Can you work these out from the model? Positions are in its coordinate system, mm. Face numbers are marked on the shaded views. A direction names the side the tool comes from. Coordinates: 2 decimals unless noted, no trailing zeros. Write each loop counter-clockwise with the first axis right and the second up, starting at its lowest first coordinate (ties: lowest second). Pieces come first, ordered by that corner, then holes.
```python
from build123d import *

# Parameters (mm, degrees)
SKETCH1_R           = 5
SKETCH1_R_2         = 1.8
BOSS_EXTRUDE1_DEPTH = 10
CHAMFER1_SIZE       = 0.5
CUT_EXTRUDE2_DEPTH  = 2.5
CHAMFER2_SIZE       = 0.5
SKETCH4_R           = 1.8
CUT_EXTRUDE3_DEPTH  = 10
CHAMFER3_SIZE       = 0.5
CHAMFER3_SIZE_2     = 0.923879533
CHAMFER3_SIZE_3     = 0.552958444
SKETCH7_R           = 10.975
SKETCH7_R_2         = 5
BOSS_EXTRUDE2_DEPTH = 15.18
SKETCH8_R           = 8.5125
CUT_EXTRUDE6_DEPTH  = 11.18
SKETCH9_R           = 9.5125
CUT_EXTRUDE8_DEPTH  = 6.32
CHAMFER4_SIZE       = 0.25


with BuildPart() as part:
    # Sketch1 → Boss-Extrude1 (new body)
    with BuildSketch(Plane.XY):
        with BuildLine():
            Line((-40.746699048, 8.183561953), (-33.214821075, -10))
            Line((-33.214821075, -10), (-9.797958971, -10))
            ThreePointArc((-9.797958971, -10), (0, -14), (9.797958971, -10))
            Line((9.797958971, -10), (19.5, -10))
            Line((19.5, -10), (19.5, -3.981225471))
            ThreePointArc((19.5, -3.981225471), (20, 4.0125), (20.5, -3.981225471))
            Line((20.5, -3.981225471), (20.5, -10))
            Line((20.5, -10), (33.214821075, -10))
            Line((33.214821075, -10), (40.746699048, 8.183561953))
            ThreePointArc((40.746699048, 8.183561953), (0, 18.25), (-40.746699048, 8.183561953))
        make_face()
        Circle(SKETCH1_R, mode=Mode.SUBTRACT)
        with Locations((-32.052211881, 8.130884627)):
            Circle(SKETCH1_R_2, mode=Mode.SUBTRACT)
        with Locations(Location((32.052211881, 8.130884627, 0), (0, 0, 180))):
            Circle(SKETCH1_R_2, mode=Mode.SUBTRACT)
        with Locations((-22, 10)):
            Circle(SKETCH1_R_2, mode=Mode.SUBTRACT)
        with Locations(Location((22, 10, 0), (0, 0, 180))):
            Circle(SKETCH1_R_2, mode=Mode.SUBTRACT)
        Polygon((-25.988511975, 6.5901118), (-35.250404289, 2.75371039), (-31.414002879, -6.508181923), (-22.152110566, -2.671780514), align=None, mode=Mode.SUBTRACT)
    extrude(amount=BOSS_EXTRUDE1_DEPTH)

    # Chamfer1
    chamfer1_edges = [part.edges().sort_by_distance(p)[0] for p in [
        (20, 4.0125, 0),
        (-24.070311271, 1.959165643, 0),
        (-30.619458132, 4.671911095, 0),
        (-33.332203584, -1.877235766, 0),
        (-26.783056723, -4.589981218, 0),
    ]]
    chamfer(chamfer1_edges, length=CHAMFER1_SIZE)

    # Sketch3 → Cut-Extrude2 (cut)
    with BuildSketch(Plane.XY.offset(3.75)):
        Polygon((-37.076762037, 12.944469155), (-33.567560961, 4.472508325), (-28.393835579, 6.615535546), (-31.903036655, 15.087496376), align=None)
        Polygon((37.076762037, 12.944469155), (33.567560961, 4.472508325), (28.393835579, 6.615535546), (31.903036655, 15.087496376), align=None)
    extrude(amount=CUT_EXTRUDE2_DEPTH, mode=Mode.SUBTRACT)

    # Chamfer2
    chamfer2_edges = [part.edges().sort_by_distance(p)[0] for p in [
        (14.648979486, -10, 0),
        (0, -14, 0),
        (-21.506390023, -10, 0),
        (-36.980760062, -0.908219024, 0),
        (0, 18.25, 0),
        (36.980760062, -0.908219024, 0),
        (26.857410538, -10, 0),
    ]]
    chamfer(chamfer2_edges, length=CHAMFER2_SIZE)

    # Sketch4 → Cut-Extrude3 (cut)
    with BuildSketch(Plane(origin=(-29.114518455, -12.059628406, 0), x_dir=(0, 0, -1), z_dir=(0.9238795325112882, 0.38268343236508634, 0))):
        with Locations(Location((-5.25, 11.021342374, 0), (0, 0, 90))):
            Circle(SKETCH4_R)
    extrude(amount=-CUT_EXTRUDE3_DEPTH, mode=Mode.SUBTRACT)

    # Chamfer3
    # the kernel refuses this chamfer: 0.923879533, 0.552958444, 0.5 mm, written as the material it takes off along each edge
    with BuildSketch(Plane(origin=(40.746699048, 8.183561953, -0.920037939), x_dir=(-0.38268343236508906, -0.923879532511287, 0), z_dir=(0, 0, 1))) as chamfer3_piece_1:
        with BuildLine():
            Line((CHAMFER3_SIZE, 0), (-0.048717445, -0.548717445))
            ThreePointArc((-0.048717445, -0.548717445), (-0.025540103, -0.282767493), (0, 0))
            Line((0, 0), (CHAMFER3_SIZE, 0))
        make_face()
    extrude(amount=12.340075878, mode=Mode.SUBTRACT)
    with BuildSketch(Plane(origin=(33.214821075, -10, -1.895315111), x_dir=(-1, 0, 0), z_dir=(0, 0, 1)), Plane(origin=(-33.214821075, -10, -1.895315111), x_dir=(-0.38268343236508656, 0.9238795325112881, 0), z_dir=(0, 0, 1))) as chamfer3_piece_2:
        Polygon((CHAMFER3_SIZE, 0), (-CHAMFER3_SIZE_2 * 0.382683432163, -CHAMFER3_SIZE_2 * 0.923879532023), (0, 0), align=None)
    extrude(amount=14.290630221, mode=Mode.SUBTRACT)
    with BuildSketch(Plane(origin=(-40.746699048, 8.183561953, -0.925350902), x_dir=(0.38268343236508684, -0.9238795325112881, 0), z_dir=(0, 0, 1))) as chamfer3_piece_3:
        with BuildLine():
            Line((CHAMFER3_SIZE_3, 0), (-0.04424113, 0.496614821))
            ThreePointArc((-0.04424113, 0.496614821), (-0.0231658, 0.256042208), (0, 0))
            Line((0, 0), (CHAMFER3_SIZE_3, 0))
        make_face()
    extrude(amount=12.350701805, mode=Mode.SUBTRACT)

    # Sketch7 → Boss-Extrude2 (add)
    with BuildSketch(Plane.XY.offset(10)):
        Circle(SKETCH7_R)
        Circle(SKETCH7_R_2, mode=Mode.SUBTRACT)
    extrude(amount=BOSS_EXTRUDE2_DEPTH)

    # Sketch8 → Cut-Extrude6 (cut)
    with BuildSketch(Plane.XY):
        with Locations(Location((0, 0, 0), (0, 0, 180))):
            Circle(SKETCH8_R)
    extrude(amount=CUT_EXTRUDE6_DEPTH, mode=Mode.SUBTRACT)

    # Sketch9 → Cut-Extrude8 (cut)
    with BuildSketch(Plane.XY):
        with Locations(Location((0, 0, 0), (0, 0, 180))):
            Circle(SKETCH9_R)
    extrude(amount=CUT_EXTRUDE8_DEPTH, mode=Mode.SUBTRACT)

    # Chamfer4
    chamfer4_edges = [part.edges().sort_by_distance(p)[0] for p in [
        (-10.975, 0, 25.18),
        (-5, 0, 25.18),
        (8.5125, 0, 6.32),
    ]]
    chamfer(chamfer4_edges, length=CHAMFER4_SIZE)


solid = part.part
```
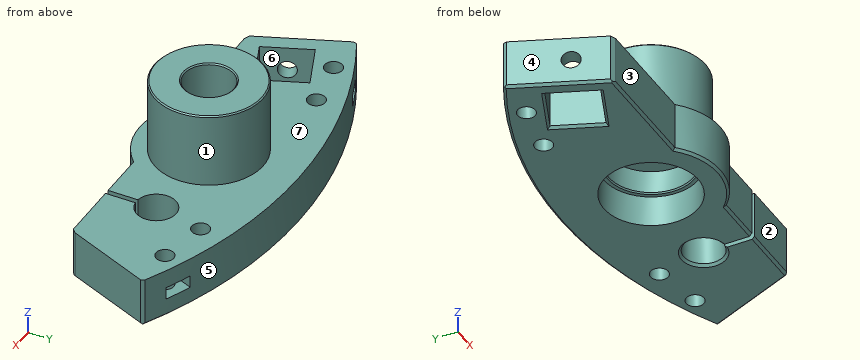
1. I'm going to push flat-ended pins straight in: P1, Ø5.5, axis at x = -3.5, y = 3.5, coming from the -Z side; P2, Ø4, axis at x = 22, y = 10, coming from the +Z side; P3, Ø10, axis at y = -4.5, z = 10, coming from the +X side. Where does each tip first touch, or does it pass through?
2. If I drill on L1, parallel to Y at x = 0, z = 23.75 (3 decimals); L2, parallel to X at y = 1, z = 7.5; L3, parallel to X at y = 0.5, z = 6.5, over which ranges is the centre line in solid material (lowest first)?
3. If we section it at C-C, the plane x = 22: Count the separate pieces of the cut face and the enclosed holes in it, plus the area to 3 significant figures.
4. Which directions (+Z, -Z, +X, -X, +Y, -Y) give clear straight access to the entire face, cutting with the end or side of a thin tool? Please do the marked faces 1, 2 and 3.
5. If we section it at B-B, the plane z = 18.75: List the corners of the cut face in (x, y) for me (3 decimals), plus the area to 3 significant figures.
6. We'd pull the mould along Y, two halves only. Please class the marked faces 4, 5, 6 and 7: released by +Y, released by -Y, zero draft, split by the parting line, or undercut.
Answers:
1. P1: stops at z = 11.18
1. P2: stops at z = 10
1. P3: stops at x = 37.56
2. L1: y = -10.975 to -5, 5 to 10.975
2. L2: x = -37.77 to -34.52, -23.67 to -8.45, 8.45 to 16.11, 23.89 to 37.77
2. L3: x = -37.56 to -34.32, -23.47 to -8.57, 8.57 to 16.02, 23.98 to 37.56
3. separate pieces: 3
3. enclosed holes: 0
3. area: 148 mm2
4. face 1: +Z
4. face 2: +Z, -Z, +X, -Y
4. face 3: +Z, -Z, -X, -Y
5. outline: circle Ø21.95 at (0, 0); hole circle Ø10 at (0, 0)
5. area: 300 mm2
6. face 4: released by -Y
6. face 5: released by +Y
6. face 6: undercut
6. face 7: zero draft
